Job drawing, mm, ordinate dimensions from the low corner. One solid piece. A direction names the side the tool comes from. Coordinates: 2 decimals unless noted, no trailing zeros. Loops run counter-clockwise (first coordinate to the right, second up) from the corner with the lowest first, then second, coordinate; pieces in that order, holes last. Notation, with made-up numbers: (77, 68) - (108, 68) arc R20 ccw to (108, 76) - close; hole circle Ø8 at (-28, 21). An arc over 180 degrees is marked (long way). Use a Markdown table: item, result. Add a question column.
1) Band-saw the part on A-A (y = 2.65). Give the cut face in (x, z) (3 decimals).
2) Band-saw the part on C-C (z = 13). Give the cut face in (x, y) (3 decimals).
3) Tool access for the marked faces 1 and 2: list every direction of +Z, -Z, +X, -X, +Y, -Y with a clear straight run to the whole face (end or side of a thin tool).
4) Probe probe 1 along Z at (x, y) = (2.4, 3.6); probe 2 along Z at (x, y) = (0.35, 2); probe 3 along Y at (x, z) = (1.45, 5.5). List the from-to ranges inside material, lowest first. Write a range as [from, to].
5) Drop flat-ended pins along their axis: P1, Ø1, axis at x = 4, z = 23, coming from the -Y side; P2, Ø1.5, axis at y = 4.5, z = 27.5, coming from the +X side; P3, Ø1, axis at x = 3, z = 24.5, coming from the -Y side; P4, Ø2, axis at x = 1, z = 10, coming from the -Y side. Give the stop position or say it passes through.
6) Band-saw the part on D-D (z = 32.5). Give the cut face in (x, y) (3 decimals), plus the area to 3 significant figures.
7) Band-saw the part on B-B (x = 2.7). Give the cut face in (y, z), plus the area to 3 significant figures.
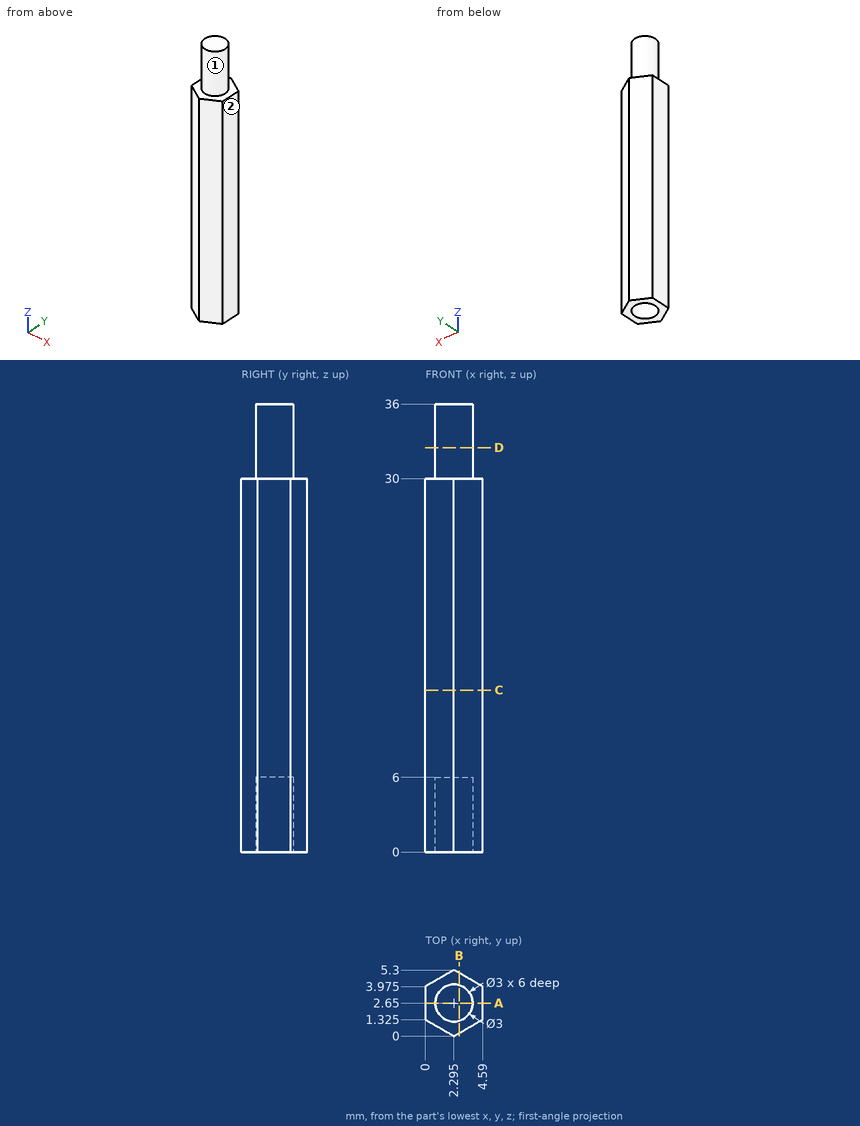
Answer block:
| question | item | result |
|---|---|---|
| 1 | outline | (0, 0) - (0.795, 0) - (0.795, 6) - (3.795, 6) - (3.795, 0) - (4.59, 0) - (4.59, 30) - (3.795, 30) - (3.795, 36) - (0.795, 36) - (0.795, 30) - (0, 30) - close |
| 2 | outline | (0, 1.325) - (2.295, 0) - (4.59, 1.325) - (4.59, 3.975) - (2.295, 5.3) - (0, 3.975) - close |
| 3 | face 1 | +Z |
| 3 | face 2 | +Z, -Z, +X, +Y, -Y |
| 4 | probe 1 | [6, 36] |
| 4 | probe 2 | [0, 30] |
| 4 | probe 3 | [0.49, 1.41], [3.89, 4.81] |
| 5 | P1 | y = 0.7 |
| 5 | P2 | x = 4.59 |
| 5 | P3 | y = 0.12 |
| 5 | P4 | y = 0.17 |
| 6 | outline | circle Ø3 at (2.295, 2.65) |
| 6 | area | 7.07 mm2 |
| 7 | outline | (0.23, 0) - (1.21, 0) - (1.21, 6) - (4.09, 6) - (4.09, 0) - (5.07, 0) - (5.07, 30) - (4.09, 30) - (4.09, 36) - (1.21, 36) - (1.21, 30) - (0.23, 30) - close |
| 7 | area | 145 mm2 |
